Could you check a few things on this model? Use its own coordinates, in mm. Face numbers are marked on the shaded views. A direction names the side the tool comes from. Round coordinates to 2 decimals unless told otherwise and drop trailing zeros. Loops run counter-clockwise (first coordinate to the right, second up) from the corner with the lowest first, then second, coordinate; pieces in that order, holes last. Notation, with made-up numbers: M 15.25,67 L 62.25,67 A19 ccw 62.25,79 Z; hole C 19.25,67.25 d8. An arc over 180 degrees is marked long. Answer in a Markdown table with one row per item.
```python
from build123d import *

# Parameters (mm, degrees)
BOSS_EXTRU_1_DEPTH      = 8
ENL_V_MAT_EXTRU_1_REACH = 124.251
ESQUISSE2_R             = 1.65
CONG_1_R                = 5
ENL_V_MAT_EXTRU_2_DEPTH = 3
CONG_2_R                = 5
CONG_3_R                = 5
CONG_4_R                = 5


with BuildPart() as part:
    # Esquisse1 → Boss.-Extru.1 (new body)
    with BuildSketch(Plane.XY):
        Polygon((0, 10.5), (0, 15.5), (50, 15.5), (50, 19.5), (71, 19.5), (71, 15.5), (121, 15.5), (121, 10.5), (121, 0), (116, 0), (116, 10.5), (105, 10.5), (105, 0), (95, 0), (95, 10.5), (71, 10.5), (71, 0), (66, 0), (66, 10.5), (66, 14.5), (55, 14.5), (55, 10.5), (55, 0), (50, 0), (50, 10.5), (26, 10.5), (26, 0), (16, 0), (16, 10.5), (5, 10.5), (5, 0), (0, 0), align=None)
    extrude(amount=BOSS_EXTRU_1_DEPTH)

    # Esquisse2 → Enlèv. mat.-Extru.1 (cut, up to next)
    with BuildSketch(Plane(origin=(0, 15.5, 0), x_dir=(1, 0, 0), z_dir=(0, 1, 0)), mode=Mode.PRIVATE) as enl_v_mat_extru_1_sk1:
        with Locations(Location((21, -4, 0), (0, 0, 270))):
            Circle(ESQUISSE2_R)
    enl_v_mat_extru_1_tool1 = extrude(enl_v_mat_extru_1_sk1.sketch, amount=-ENL_V_MAT_EXTRU_1_REACH, mode=Mode.PRIVATE) & part.part
    # Esquisse2 → Enlèv. mat.-Extru.1 (cut, up to next)
    with BuildSketch(Plane(origin=(0, 15.5, 0), x_dir=(1, 0, 0), z_dir=(0, 1, 0)), mode=Mode.PRIVATE) as enl_v_mat_extru_1_sk2:
        with Locations(Location((100, -4, 0), (0, 0, 270))):
            Circle(ESQUISSE2_R)
    enl_v_mat_extru_1_tool2 = extrude(enl_v_mat_extru_1_sk2.sketch, amount=-ENL_V_MAT_EXTRU_1_REACH, mode=Mode.PRIVATE) & part.part
    add(enl_v_mat_extru_1_tool1.solids().sort_by_distance((21, 15.5, 4))[0], mode=Mode.SUBTRACT)
    add(enl_v_mat_extru_1_tool2.solids().sort_by_distance((100, 15.5, 4))[0], mode=Mode.SUBTRACT)

    # Congé1
    # the kernel refuses this fillet: 5 mm, written as the material it takes off along each edge
    with BuildSketch(Plane(origin=(50, 19.5, -12.247448714), x_dir=(1.568523089189919e-12, -1.0, 0), z_dir=(0, 0, 1))) as cong_1_piece_1:
        with BuildLine():
            CenterArc((5, 4.898979486), CONG_1_R, 180, 78.463040967)
            Line((0, 4.898979486), (-0.1, 4.898979486))
            Line((-0.1, 4.898979486), (-0.1, 0))
            Line((-0.1, 0), (0, -0.1))
            ThreePointArc((0, -0.1), (2, -0.1), (3.98, -0.09797959))
            Line((3.98, -0.09797959), (4, 0))
        make_face()
    extrude(amount=32.494897428, mode=Mode.SUBTRACT)
    with BuildSketch(Plane(origin=(71, 19.5, -12.247448714), x_dir=(-1, 0, 0), z_dir=(0, 0, 1))) as cong_1_piece_2:
        with BuildLine():
            CenterArc((4.898979486, 5), CONG_1_R, 191.536959033, 78.463040967)
            Line((0, 4), (-0.09797959, 3.98))
            ThreePointArc((-0.09797959, 3.98), (-0.1, 2), (-0.1, 0))
            Line((-0.1, 0), (0, -0.1))
            Line((0, -0.1), (4.898979486, -0.1))
            Line((4.898979486, -0.1), (4.898979486, 0))
        make_face()
    extrude(amount=32.494897428, mode=Mode.SUBTRACT)

    # Esquisse3 → Enlèv. mat.-Extru.2 (cut)
    with BuildSketch(Plane(origin=(0, 15.5, 0), x_dir=(1, 0, 0), z_dir=(0, 1, 0))):
        Polygon((19.354551733, -1.15), (22.645448267, -1.15), (24.290896534, -4), (22.645448267, -6.85), (19.354551733, -6.85), (17.709103466, -4), align=None)
        Polygon((103.290896534, -4), (101.645448267, -1.15), (98.354551733, -1.15), (96.709103466, -4), (98.354551733, -6.85), (101.645448267, -6.85), align=None)
    extrude(amount=-ENL_V_MAT_EXTRU_2_DEPTH, mode=Mode.SUBTRACT)

    # Congé2
    cong_2_edges = [part.edges().sort_by_distance(p)[0] for p in [
        (0, 15.5, 4),
        (121, 15.5, 4),
    ]]
    fillet(cong_2_edges, radius=CONG_2_R)

    # Congé3
    cong_3_edges = [part.edges().sort_by_distance(p)[0] for p in [
        (95, 10.5, 4),
        (71, 10.5, 4),
        (50, 10.5, 4),
        (26, 10.5, 4),
    ]]
    fillet(cong_3_edges, radius=CONG_3_R)

    # Congé4
    cong_4_edges = [part.edges().sort_by_distance(p)[0] for p in [
        (50, 15.5, 4),
        (71, 15.5, 4),
    ]]
    fillet(cong_4_edges, radius=CONG_4_R)


solid = part.part
```
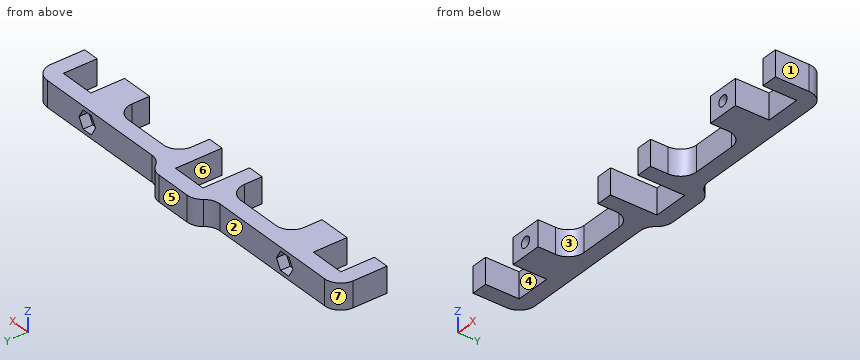
1) I want a section at B-B, the plane y = 2. Please give me the cut outline in (x, z).
Computed:
| item | result |
|---|---|
| outline | M 0,0 L 5,0 L 5,8 L 0,8 Z; M 16,0 L 26,0 L 26,8 L 16,8 Z; M 50,0 L 55,0 L 55,8 L 50,8 Z; M 66,0 L 71,0 L 71,8 L 66,8 Z; M 95,0 L 105,0 L 105,8 L 95,8 Z; M 116,0 L 121,0 L 121,8 L 116,8 Z; hole C 21,4 d3.3; hole C 100,4 d3.3 |
2) If we mould it in two halves opening along X, with no side actions, what happens to the marked faces 4, 5, 6 and 7? For each: released by +X, released by -X, zero draft, split by the parting line, or undercut.
Computed:
| item | result |
|---|---|
| face 4 | undercut |
| face 5 | zero draft |
| face 6 | undercut |
| face 7 | released by -X |
3) I want a section at C-C, the plane x = 57.5. Please give me the cut outline in (y, z).
Computed:
| item | result |
|---|---|
| outline | M 14.5,0 L 19.5,0 L 19.5,8 L 14.5,8 Z |
4) Will these pins go through, and if not, where does the flat tip stop? P1, Ø3, axis at x = 22.5, z = 2.5, coming from the +Y side; P2, Ø4, axis at x = 31.5, z = 3, coming from the -Y side; P3, Ø2.5, axis at x = 108, z = 5.5, coming from the -Y side.
Computed:
| item | result |
|---|---|
| P1 | stops at y = 15.5 |
| P2 | stops at y = 10.27 |
| P3 | stops at y = 10.5 |
5) Which directions (+Z, -Z, +X, -X, +Y, -Y) give clear straight access to the entire face, cutting with the end or side of a thin tool? Please do the marked faces 1, 2 and 3.
Computed:
| item | result |
|---|---|
| face 1 | +Z, -Z, +X, +Y, -Y |
| face 2 | +Z, -Z, -X, +Y |
| face 3 | +Z, -Z, -Y |
6) I want a section at A-A, the plane x = 21. Please give me the cut outline in (y, z), plus the area to 4 significant figures.
Computed:
| item | result |
|---|---|
| outline | M 0,0 L 15.5,0 L 15.5,1.15 L 12.5,1.15 L 12.5,2.35 L 0,2.35 Z; M 0,5.65 L 12.5,5.65 L 12.5,6.85 L 15.5,6.85 L 15.5,8 L 0,8 Z |
| area | 65.65 mm² |
7) I need wall thicknesses on line 1 (X direction, y = 3.5, z = 6); line 2 (Z direction, x = 100, y = 6.5); line 3 (X direction, y = 7.75, z = 6.5). Which ranges of each line are inside material? Lowest first, please.
Computed:
| item | result |
|---|---|
| line 1 | x = 0 to 5, 16 to 26, 50 to 55, 66 to 71, 95 to 105, 116 to 121 |
| line 2 | z = 0 to 2.35, 5.65 to 8 |
| line 3 | x = 0 to 5, 16 to 26.53, 49.47 to 55, 66 to 71.53, 94.47 to 105, 116 to 121 |
